from build123d import *

# Parameters (mm, degrees)
F1_DEPTH = 2
F2_R     = 1
F3_SIZE  = 0.5


with BuildPart() as f1:
    # F0 (on Top) → F1 (new body)
    with BuildSketch(Plane.XY):
        with BuildLine():
            Line((-13.294905, 21.65575), (-15.497596, 34.147833))
            ThreePointArc((-15.497596, 34.147833), (-32.475953, 18.75), (-37.321689, -3.652605))
            Line((-37.321689, -3.652605), (-25.401882, 0.68585))
            ThreePointArc((-25.401882, 0.68585), (-9.093267, -5.25), (-12.106977, -22.3416))
            Line((-12.106977, -22.3416), (-21.824093, -30.495229))
            ThreePointArc((-21.824093, -30.495229), (0.445759, -37.497351), (22.542862, -29.967806))
            Line((22.542862, -29.967806), (12.634663, -22.047478))
            ThreePointArc((12.634663, -22.047478), (9.215501, -5.03235), (25.378399, 1.289513))
            Line((25.378399, 1.289513), (37.397972, -2.764357))
            ThreePointArc((37.397972, -2.764357), (32.250779, 19.134714), (15.497596, 34.147833))
            Line((15.497596, 34.147833), (13.294905, 21.65575))
            ThreePointArc((13.294905, 21.65575), (0, 10.5), (-13.294905, 21.65575))
        make_face()
        with BuildLine():
            ThreePointArc((4.426906, 4.05), (0, -6), (-4.426906, 4.05))
            Line((-4.426906, 4.05), (4.426906, 4.05))
        make_face(mode=Mode.SUBTRACT)
    extrude(amount=F1_DEPTH)

    # F2
    f2_edges = [f1.edges().sort_by_distance(p)[0] for p in [
        (22.542862, -29.967806, 1),
        (37.397972, -2.764357, 1),
        (-21.824093, -30.495229, 1),
        (-37.321689, -3.652605, 1),
        (-15.497596, 34.147833, 1),
        (15.497596, 34.147833, 1),
    ]]
    fillet(f2_edges, radius=F2_R)

    # F3
    f3_edges = [f1.edges().sort_by_distance(p)[0] for p in [
        (30.766032, -0.527587, 0),
        (37.040868, -2.220421, 0),
        (9.215501, -5.03235, 0),
        (32.250779, 19.134714, 0),
        (17.075898, -25.597672, 0),
        (15.80384, 33.573722, 0),
        (21.89221, -29.961431, 0),
        (14.282235, 27.25518, 0),
        (0.445759, -37.497351, 0),
        (0, 10.5, 0),
        (-21.173776, -30.473388, 0),
        (-14.282235, 27.25518, 0),
        (-16.462561, -25.996369, 0),
        (-15.80384, 33.573722, 0),
        (-9.093267, -5.25, 0),
        (-32.475953, 18.75, 0),
        (-30.744796, -1.258811, 0),
        (-36.977617, -3.100334, 0),
        (0, -6, 0),
        (0, 4.05, 0),
    ]]
    chamfer(f3_edges, length=F3_SIZE)


solid = f1.part
Work out the finished part from the listing and answer in its coordinate system (mm). A direction names the side the tool comes from. Round coordinates to 2 decimals unless told otherwise and drop trailing zeros. Order: outer loops, then holes, each group sorted by start corner. A loop starts at its lowest first (then second) coordinate and runs counter-clockwise, first axis right, second up. Notation, with made-up numbers: M 18.25,-23.75 L 58.25,-23.75 A17 cw 58.25,3.25 Z; hole C 24,48.25 d7. An arc over 180 degrees is marked long. Put each result on its own line as item: value. Start each with the question number.
Q1. Section B-B, the plane z = 1.1 is taken. Write down the section's boundary in (x, y).
Q2. A flat-ended cylindrical pin translates along its axis: pin 1 (0.8 mm diameter, centred on x = 1.5, z = 1.5, fed in from -Y). Find the tip coordinate at first contact, or state that the pin passes through.
Q3. For a pull along X with two mould halves and no side action, classify faces 6 (the flat face through (14.54, 27.29, 0.25)), 7 (the conical face through (-9.11, -4.95, 0.36)), 8 (the cylindrical face through (0.1, -37.5, 1.2)), 9 (the flat face through (17.14, -25.65, 1.24)) as pulls with the +X half, pulls with the -X half, needs draft (parallel to the pull), parting line crosses it, or undercut.
Q4. Straight lines are drawn through the part: L1, parallel to Y at x = 0, z = 1.1; L2, parallel to X at y = 19.5, z = 1.35; L3, parallel to X at y = 23.5, z = 0.35. For each, find the intervals that lie inside material, in ascending order. Write a range as [from, to].
Q5. Section A-A, the plane x = 0 is taken. Write down the section's boundary in (y, z), and give its area (3 significant figures).
Q6. A tool of negligible diameter and unlimited length cuts with its end or side. For faces 1 (the flat face through (30.769, -0.269, 0.254)), 2 (the flat face through (30.69, -0.5, 1.24)), 3 (the flat face through (-14.27, 27.18, 1.24)), 4 (the flat face through (-14.511, 27.134, 0.253)), 5 (the flat face through (-16.402, -25.945, 1.24)), from which of +Z, -Z, +X, -X, +Y, -Y can it reach the whole face along a straight path? Write none if from no direction.
Findings below:
1. outline: M -37.43,-2.33 A1 ccw -36.09,-3.2 L -25.4,0.69 A13.5 cw -12.11,-22.34 L -20.82,-29.65 A1 ccw -20.73,-31.25 A37.5 ccw 21.47,-30.75 A1 ccw 21.52,-29.15 L 12.63,-22.05 A13.5 cw 25.38,1.29 L 36.15,-2.34 A1 ccw 37.47,-1.44 A37.5 ccw 16.7,33.58 A1 ccw 15.27,32.85 L 13.29,21.66 A13.5 cw -13.29,21.66 L -15.27,32.85 A1 ccw -16.7,33.58 A37.5 ccw Z; hole M -4.43,4.05 A6 ccw long 4.43,4.05 Z
2. pin 1: stops at y = -37.48
3. face 6: undercut
3. face 7: undercut
3. face 8: parting line crosses it
3. face 9: pulls with the +X half
4. L1: y = [-37.5, -6], [4.05, 10.5]
4. L2: x = [-32.03, -12.73], [12.73, 32.03]
4. L3: x = [-29.03, -13.77], [13.77, 29.03]
5. outline: M -37.5,0.5 L -37,0 L -6.5,0 L -6,0.5 L -6,2 L -37.5,2 Z; M 4.05,0.5 L 4.55,0 L 10,0 L 10.5,0.5 L 10.5,2 L 4.05,2 Z
5. area: 75.4 mm^2
6. face 1: -Z, -Y
6. face 2: +Z, -Z, -Y
6. face 3: +Z, -Z, +Y
6. face 4: -Z, +Y
6. face 5: +Z, -Z, -X
